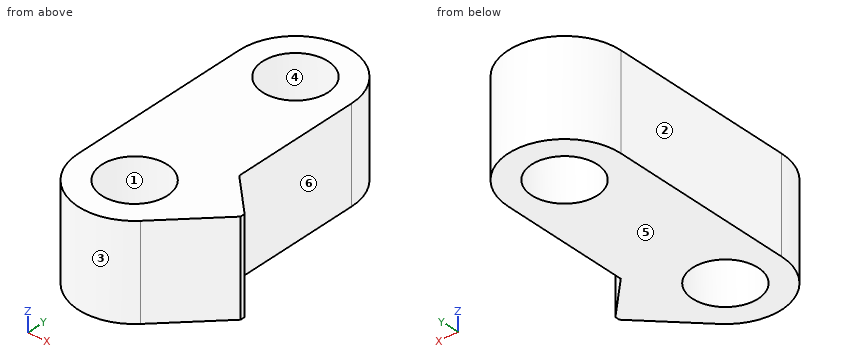
Autodesk Inventor part; units mm, degrees
ref_plane "YZ Plane" through (0, 0, 0) normal (1, 0, 0) x (0, 1, 0)
ref_plane "XZ Plane" through (0, 0, 0) normal (0, 1, 0) x (-1, 0, 0)
ref_plane "XY Plane" through (0, 0, 0) normal (0, 0, 1) x (1, 0, 0)
sketch "Sketch1" plane through (0, 0, 0) normal (0, 0, 1) x (1, 0, 0)
  circle A0 centre (0, 0) radius 1.75
  circle A1 centre (0, -10) radius 1.75
  arc A2 (-3, -10) -> (3, -10) centre (0, -10) ccw
  arc A3 (3, 0) -> (-3, 0) centre (0, 0) ccw
  line L0 (-3, -10) -> (-3, 0)
  line L1 (3, -10) -> (3, 0)
  line L2 (2.1213, -12.1213) -> (5, -9.2426)
  line L3 (2.1213, -12.1213) -> (4.3055, -12.1213) construction
  line L4 (5, -9.2426) -> (5, -8.9926)
  line L5 (5, -8.9926) -> (3, -6.9926)
  point P0 (3, -7.757)
  dimension "d0" = 3.5
  dimension "d1" = 3.5
  dimension "d2" = 6
  dimension "d3" = 6
  dimension "d6" = 45
  dimension "d10" = 5
  dimension "d11" = 0.25
  dimension "d12" = 135
extrude "Extrusion1" add sketch "Sketch1" along normal blind 5
properties part number "mellemStykke"
Here's how the part is built. I have some questions about the finished solid (model axes, mm). Face numbers are marked on the shaded views. A direction names the side the tool comes from. Coordinates: 2 decimals unless noted, no trailing zeros. Order: outer loops, then holes, each group sorted by start corner. A loop starts at its lowest first (then second) coordinate and runs counter-clockwise, first axis right, second up. Notation, with made-up numbers: M 41,84.25 L 62,84.25 A20 cw 62,116.25 Z; hole C -35,-38 d2. An arc over 180 degrees is marked long. Answer as a JSON object with one key per item and string values. Group by question number.
(1) Which directions (+Z, -Z, +X, -X, +Y, -Y) give clear straight access to the entire face, cutting with the end or side of a thin tool? Please do the marked faces 5 and 6.
(2) If we mould it in two halves opening along Y, with no side actions, what happens to the marked faces 1, 2, 3 and 4? For each: released by +Y, released by -Y, zero draft, split by the parting line, or undercut.
(3) For pin 1 (1 mm diameter, centred on y = -11.5, z = 0.5, fed in from -X), with a flat end and sliding along its axis, tell me the tip position at first contact or that it passes through.
(4) Suppose I cut it at A-A, the plane x = 0. Please give me the cut outline in (y, z), then the cut area to 3 significant figures.
(5) I need wall thicknesses on probe 1 along Y at (x, z) = (0, 3); probe 2 along Y at (x, z) = (-1, 3.8); probe 3 along X at (y, z) = (-3.5, 3.8). Which ranges of each line are inside material? Lowest first, please.
(6) Suppose I cut it at B-B, the plane z = 2.6. Please give me the cut outline in (x, y).
(7) Suppose I cut it at C-C, the plane y = -1. Please give me the cut outline in (x, z).
(8) Suppose I cut it at D-D, the plane x = -1. Please give me the cut outline in (y, z), then the cut area to 3 significant figures.
Values found:
{
 "1": {"face 5": "-Z, +X, -X, +Y, -Y", "face 6": "+Z, -Z, +X, +Y"},
 "2": {"face 1": "undercut", "face 2": "zero draft", "face 3": "released by -Y", "face 4": "undercut"},
 "3": {"pin 1": "stops at x = -2.83"},
 "4": {"outline": "M -13,0 L -11.75,0 L -11.75,5 L -13,5 Z; M -8.25,0 L -1.75,0 L -1.75,5 L -8.25,5 Z; M 1.75,0 L 3,0 L 3,5 L 1.75,5 Z", "area": "45.0 mm^2"},
 "5": {"probe 1": "y = -13 to -11.75, -8.25 to -1.75, 1.75 to 3", "probe 2": "y = -12.83 to -11.44, -8.56 to -1.44, 1.44 to 2.83", "probe 3": "x = -3 to 3"},
 "6": {"outline": "M -3,-10 A3 ccw 2.12,-12.12 L 5,-9.24 L 5,-8.99 L 3,-6.99 L 3,0 A3 ccw -3,0 Z; hole C 0,-10 d3.5; hole C 0,0 d3.5"},
 "7": {"outline": "M -3,0 L -1.44,0 L -1.44,5 L -3,5 Z; M 1.44,0 L 3,0 L 3,5 L 1.44,5 Z"},
 "8": {"outline": "M -12.83,0 L -11.44,0 L -11.44,5 L -12.83,5 Z; M -8.56,0 L -1.44,0 L -1.44,5 L -8.56,5 Z; M 1.44,0 L 2.83,0 L 2.83,5 L 1.44,5 Z", "area": "49.6 mm^2"}
}
